Geometry check sheet. Reference: the model listing, model coordinates, mm. A direction names the side the tool comes from. Round coordinates to 2 decimals unless told otherwise and drop trailing zeros. Loops run counter-clockwise (first coordinate to the right, second up) from the corner with the lowest first, then second, coordinate; pieces in that order, holes last. Notation, with made-up numbers: (56, 76) - (109, 76) arc R10 ccw to (109, 89) - close; hole circle Ø3 at (29.25, 86). An arc over 180 degrees is marked (long way). Answer in a Markdown table with one row per item. Add a question column.
```python
from build123d import *

# Parameters (mm, degrees)
SKETCH1_R               = 10
BOSS_EXTRUDE1_DEPTH     = 150
SKETCH2_R               = 8.5
SKETCH2_R_2             = 4.5
BOSS_EXTRUDE2_DEPTH     = 14.5
CUT_EXTRUDE1_DEPTH      = 14.5
CUT_EXTRUDE1_DEPTH_BACK = 14.5
SKETCH3_R               = 1.6
SKETCH5_R               = 16
BOSS_EXTRUDE3_DEPTH     = 2.5
FILLET1_R               = 10
CUT_EXTRUDE2_DEPTH      = 2.5
SKETCH6_R               = 3
SKETCH6_R_2             = 2.5
CUT_EXTRUDE3_DEPTH      = 1


with BuildPart() as part:
    # Sketch1 → Boss-Extrude1 (new body)
    with BuildSketch(Plane(origin=(0, 0, 0), x_dir=(1, 0, 0), z_dir=(0, 1, 0))):
        with Locations(Location((0, 0, 0), (0, 0, 270))):
            Circle(SKETCH1_R)
    extrude(amount=BOSS_EXTRUDE1_DEPTH)

    # Sketch2 → Boss-Extrude2 (add)
    with BuildSketch(Plane.XZ):
        with Locations(Location((0, 0, 0), (0, 0, 90))):
            Circle(SKETCH2_R)
        with Locations(Location((0, 0, 0), (0, 0, 90))):
            Circle(SKETCH2_R_2, mode=Mode.SUBTRACT)
    extrude(amount=BOSS_EXTRUDE2_DEPTH)

    # Sketch3 → Cut-Extrude1 (cut, two sides: drawn at the far end of the back side and taken through both)
    with BuildSketch(Plane(origin=(0, 0, 0), x_dir=(0, 0, -1), z_dir=(1, 0, 0)).offset(-CUT_EXTRUDE1_DEPTH_BACK)):
        with Locations(Location((0, -7.25, 0), (0, 0, 180))):
            Circle(SKETCH3_R)
    extrude(amount=CUT_EXTRUDE1_DEPTH + CUT_EXTRUDE1_DEPTH_BACK, mode=Mode.SUBTRACT)

    # Sketch5 → Boss-Extrude3 (add)
    with BuildSketch(Plane(origin=(0, 150, 0), x_dir=(1, 0, 0), z_dir=(0, 1, 0))):
        with Locations(Location((0, 0, 0), (0, 0, 270))):
            Circle(SKETCH5_R)
    extrude(amount=-BOSS_EXTRUDE3_DEPTH)

    # Fillet1
    # the kernel refuses this fillet: 10 mm, written as the material it adds along each edge
    with BuildSketch(Plane(origin=(0, 147.5, 0), x_dir=(0, 0, 1), z_dir=(1, 0, 0))) as fillet1_piece_1:
        with BuildLine():
            CenterArc((20, 9.16515139), FILLET1_R, 180, 66.421821522)
            Line((16, 0), (15.92, -0.183303028))
            ThreePointArc((15.92, -0.183303028), (13, -0.2), (10, -0.2))
            Line((10, -0.2), (9.8, 0))
            Line((9.8, 0), (9.8, 9.16515139))
            Line((9.8, 9.16515139), (10, 9.16515139))
        make_face()
    revolve(axis=Axis((0, 147.5, 0), (0, -1, 0)))

    # Sketch4 → Cut-Extrude2 (cut)
    with BuildSketch(Plane(origin=(0, 150, 0), x_dir=(1, 0, 0), z_dir=(0, 1, 0))):
        with BuildLine():
            ThreePointArc((-11.5, 2.5), (-13.267766953, 1.767766953), (-14, 0))
            Line((-14, 0), (-9, 0))
            ThreePointArc((-9, 0), (-9.732233047, 1.767766953), (-11.5, 2.5))
        make_face()
        with BuildLine():
            Line((-9, 0), (-14, 0))
            ThreePointArc((-14, 0), (-13.267766953, -1.767766953), (-11.5, -2.5))
            ThreePointArc((-11.5, -2.5), (-9.732233047, -1.767766953), (-9, 0))
        make_face()
        with BuildLine():
            Line((-3.75, 0), (-9, 0))
            ThreePointArc((-9, 0), (-9.732233047, -1.767766953), (-11.5, -2.5))
            Line((-11.5, -2.5), (-0.805698272, -3.662424101))
            ThreePointArc((-0.805698272, -3.662424101), (-2.922658766, -2.349588419), (-3.75, 0))
        make_face()
        with BuildLine():
            ThreePointArc((-11.5, 2.5), (-9.732233047, 1.767766953), (-9, 0))
            Line((-9, 0), (-3.75, 0))
            ThreePointArc((-3.75, 0), (-2.922658766, 2.349588419), (-0.805698272, 3.662424101))
            Line((-0.805698272, 3.662424101), (-11.5, 2.5))
        make_face()
        with BuildLine():
            ThreePointArc((-0.805698272, 3.662424101), (-2.922658766, 2.349588419), (-3.75, 0))
            Line((-3.75, 0), (0, 0))
            Line((0, 0), (0, 3.75))
            Line((0, 3.75), (-0.805698272, 3.662424101))
        make_face()
        with BuildLine():
            Line((0, 0), (-3.75, 0))
            ThreePointArc((-3.75, 0), (-2.922658766, -2.349588419), (-0.805698272, -3.662424101))
            Line((-0.805698272, -3.662424101), (0, -3.75))
            Line((0, -3.75), (0.805698272, -3.662424101))
            ThreePointArc((0.805698272, -3.662424101), (2.922658766, -2.349588419), (3.75, 0))
            Line((3.75, 0), (0, 0))
        make_face()
        with BuildLine():
            Line((0, 3.75), (0, 0))
            Line((0, 0), (3.75, 0))
            ThreePointArc((3.75, 0), (2.922658766, 2.349588419), (0.805698272, 3.662424101))
            Line((0.805698272, 3.662424101), (0, 3.75))
        make_face()
        with BuildLine():
            ThreePointArc((0.805698272, 3.662424101), (2.922658766, 2.349588419), (3.75, 0))
            Line((3.75, 0), (9, 0))
            ThreePointArc((9, 0), (9.732233047, 1.767766953), (11.5, 2.5))
            Line((11.5, 2.5), (0.805698272, 3.662424101))
        make_face()
        with BuildLine():
            Line((9, 0), (3.75, 0))
            ThreePointArc((3.75, 0), (2.922658766, -2.349588419), (0.805698272, -3.662424101))
            Line((0.805698272, -3.662424101), (11.5, -2.5))
            ThreePointArc((11.5, -2.5), (9.732233047, -1.767766953), (9, 0))
        make_face()
        with BuildLine():
            ThreePointArc((11.5, 2.5), (9.732233047, 1.767766953), (9, 0))
            Line((9, 0), (11.5, 0))
            Line((11.5, 0), (11.5, 2.5))
        make_face()
        with BuildLine():
            Line((11.5, 0), (9, 0))
            ThreePointArc((9, 0), (9.732233047, -1.767766953), (11.5, -2.5))
            Line((11.5, -2.5), (11.5, 0))
        make_face()
        with BuildLine():
            ThreePointArc((14, 0), (13.267766953, 1.767766953), (11.5, 2.5))
            Line((11.5, 2.5), (11.5, 0))
            Line((11.5, 0), (14, 0))
        make_face()
        with BuildLine():
            Line((11.5, 0), (11.5, -2.5))
            ThreePointArc((11.5, -2.5), (13.267766953, -1.767766953), (14, 0))
            Line((14, 0), (11.5, 0))
        make_face()
    extrude(amount=-CUT_EXTRUDE2_DEPTH, mode=Mode.SUBTRACT)

    # Sketch6 → Cut-Extrude3 (cut)
    with BuildSketch(Plane(origin=(0, 147.5, 0), x_dir=(1, 0, 0), z_dir=(0, 1, 0))):
        with Locations(Location((0, 0, 0), (0, 0, 270))):
            Circle(SKETCH6_R)
        with Locations(Location((0, 0, 0), (0, 0, 270))):
            Circle(SKETCH6_R_2, mode=Mode.SUBTRACT)
    extrude(amount=-CUT_EXTRUDE3_DEPTH, mode=Mode.SUBTRACT)


solid = part.part
```
Q1. Cross-section at A-A, the plane y = -7.25. Enter the section's corners in (x, z), plus the area to 3 significant figures.
Q2. Scan lines: line 1 (Y direction, x = -5.55, z = 0); line 2 (Y direction, x = 5, z = -8); line 3 (Z direction, x = -3, y = -1.5). Record each from-to range of solid material in increasing order. Write a range as from..to.
Q3. Set-up check for faces 1 (the cylindrical face through (-9.76, 68.2, -2.17)), 2 (the cylindrical face through (0.9, 147.01, 2.86)), 3 (the flat face through (0, 150, -4)): record each of +Z, -Z, +X, -X, +Y, -Y from which the full face is reachable in a straight line by a thin tool's end or side.
Q4. Release check for a two-part mould opening along X. For faces 4 (the cylindrical face through (8.3, -7.15, -1.84)), 5 (the flat face through (-7.4, 0, -4.5)), 6 (the flat face through (0, 0, 0)) record: +X half, -X half, draft (parallel to the pull), parting line (faces both ways), or undercut.
Q5. Depth check by flat-ended pin: P1, Ø3, axis at y = 19.5, z = -1.5, coming from the -X side; P2, Ø3, axis at x = 1.5, z = 0.5, coming from the +Y side; P3, Ø4, axis at x = -2, z = -11.5, coming from the -Y side. Enter the tip coordinate at first touch or a pass-through.
Q6. Cross-section at B-B, the plane y = 53. Enter the section's corners in (x, z).
Check sheet entries:
| question | item | result |
|---|---|---|
| 1 | outline | (-8.35, -1.6) arc R8.5 ccw to (8.35, -1.6) - (4.21, -1.6) arc R4.5 cw to (-4.21, -1.6) - close; (-8.35, 1.6) - (-4.21, 1.6) arc R4.5 cw to (4.21, 1.6) - (8.35, 1.6) arc R8.5 ccw to start |
| 1 | area | 137 mm² |
| 2 | line 1 | -14.5..-8.85, -5.65..147.5 |
| 2 | line 2 | 0..150 |
| 2 | line 3 | -7.95..-3.35, 3.35..7.95 |
| 3 | face 1 | -Y |
| 3 | face 2 | +Y |
| 3 | face 3 | +Z, -Z, +X, -X, +Y |
| 4 | face 4 | parting line |
| 4 | face 5 | draft |
| 4 | face 6 | undercut |
| 5 | P1 | x = -10 |
| 5 | P2 | y = 147.5 |
| 5 | P3 | y = 0 |
| 6 | outline | circle Ø20 at (0, 0) |
